Source: CAD feature listing. Evaluate the final solid. Frame: model axes, mm. Face numbers are marked on the shaded views. A direction names the side the tool comes from. Give positions to 0.01 mm unless a question says otherwise; leave off trailing zeros. Loops run counter-clockwise (first coordinate to the right, second up) from the corner with the lowest first, then second, coordinate; pieces in that order, holes last. Notation, with made-up numbers: (-14.75, 12) - (35.25, 12) arc R32 ccw to (35.25, 49) - close; hole circle Ø8 at (-17, 59). An arc over 180 degrees is marked (long way). Put each result on its own line as item: value.
Autodesk Fusion 360 part; units mm, degrees
sketch "Sketch1" plane through (0, 0, 0) normal (0, 0, 1) x (1, 0, 0) in component "pretensioner"
  line L0 (10, 0) -> (20, 0)
  line L1 (20, 0) -> (20, 42)
  line L2 (20, 42) -> (0, 42)
  line L3 (0, 42) -> (0, 22)
  line L4 (0, 42) -> (20, 42) construction
  line L5 (20, 42) -> (20, 22) construction
  line L6 (20, 22) -> (0, 22) construction
  line L7 (0, 22) -> (0, 42) construction
  circle A0 centre (10, 32) radius 3
  line L8 (10, 22) -> (10, 0)
  line L9 (10, 0) -> (20, 0)
  line L10 (20, 0) -> (20, 22)
  line L11 (10, 22) -> (0, 22)
  dimension "d1" = 20
  dimension "d2" = 42
  dimension "d3" = 20
  dimension "d4" = 6
  dimension "d5" = 10
extrude "Extrude1" add sketch "Sketch1" along normal blind 4.3 in component "pretensioner"
component "pretensioner" placed x (1, 0, 0) y (0, 1, 0) z (0, 0, 1) at (0, 0, 0)
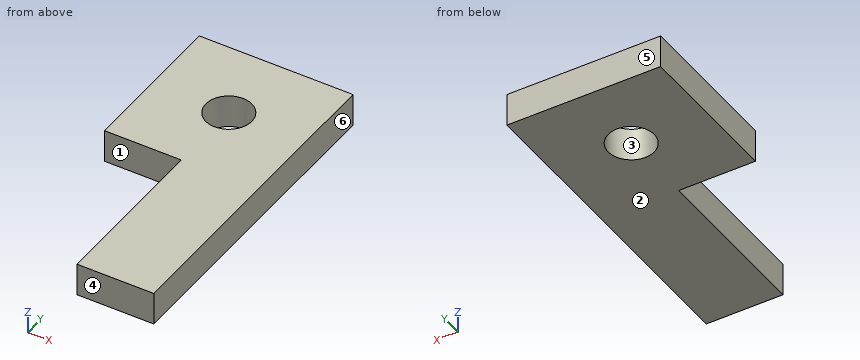
1) Material intervals for line 1 along X through (y, z) = (10, 3.05); line 2 along Y through (x, z) = (2.5, 4.15); line 3 along X through (y, z) = (30.5, 1.8), sorted ascending. Write a range as [from, to].
Check result:
line 1: [10, 20]
line 2: [22, 42]
line 3: [0, 7.4], [12.6, 20]
2) Section query A-A, the plane y = 32. Output: boundary loops of the cut face in (x, z), plus the area to 3 significant figures.
Check result:
outline: (0, 0) - (7, 0) - (7, 4.3) - (0, 4.3) - close; (13, 0) - (20, 0) - (20, 4.3) - (13, 4.3) - close
area: 60.2 mm²
3) Pin query (flat end, axial travel): P1, Ø9.5, axis at x = 10, y = 32, coming from the -Z side; P2, Ø1, axis at x = 7, y = 20.5, coming from the +Z side; P3, Ø2, axis at y = 9.5, z = 1.5, coming from the -X side; P4, Ø1.3, axis at x = 3.5, z = 2.5, coming from the -Y side. Return the tip coordinate at first contact, or that it passes through.
Check result:
P1: z = 0
P2: through
P3: x = 10
P4: y = 22
4) Mould query, pull axis Y, two halves, no side actions, for the marked faces 3, 4, 5 and 6. Classes: pulls with the +Y half, pulls with the -Y half, needs draft (parallel to the pull), parting line crosses it, or undercut.
Check result:
face 3: undercut
face 4: pulls with the -Y half
face 5: pulls with the +Y half
face 6: needs draft
5) Section query C-C, the plane x = 3.5. Output: boundary loops of the cut face in (y, z), plus the area to 3 significant figures.
Check result:
outline: (22, 0) - (42, 0) - (42, 4.3) - (22, 4.3) - close
area: 86.0 mm²
6) Section query B-B, the plane z = 0.6. Output: boundary loops of the cut face in (x, y).
Check result:
outline: (0, 22) - (10, 22) - (10, 0) - (20, 0) - (20, 42) - (0, 42) - close; hole circle Ø6 at (10, 32)
7) Access query for the marked faces 1 and 2. Directions: +Z, -Z, +X, -X, +Y, -Y. A direction counts if a zero-diameter tool reaches every point of the face in a straight line with its end or side. Return the directions, or none.
Check result:
face 1: +Z, -Z, -X, -Y
face 2: -Z, +X, -X, +Y, -Y
8) Section query D-D, the plane y = 8. Output: boundary loops of the cut face in (x, z).
Check result:
outline: (10, 0) - (20, 0) - (20, 4.3) - (10, 4.3) - close
